from build123d import *

# Parameters (mm, degrees)
F2_R     = 0.4
F3_SIZE2 = 0.3
F3_SIZE  = 1


with BuildPart() as f1:
    # F0 (on Right) → F1 (revolve)
    with BuildSketch(Plane.YZ):
        Polygon((1.5, 15.5), (0, 15.5), (0, 10), (16.5, 10), (16.5, 11.5), (1.5, 11.5), align=None)
    revolve(axis=Axis((0, 9.5578194596, 0), (0, 1, 0)))

    # F2
    f2_edges = [f1.edges().sort_by_distance(p)[0] for p in [
        (0, 0, -10),
    ]]
    fillet(f2_edges, radius=F2_R)

    # F3
    f3_edges = [f1.edges().sort_by_distance(p)[0] for p in [
        (0, 16.5, -11.5),
    ]]
    f3_side = f1.faces().sort_by_distance((0, 9, -11.5))[0]
    chamfer(f3_edges, length=F3_SIZE, length2=F3_SIZE2, reference=f3_side)


solid = f1.part
For this review, take the finished solid that the model builds, in its own axes (mm). Round coordinates to 2 decimals unless told otherwise and drop trailing zeros. Order: outer loops, then holes, each group sorted by start corner. A loop starts at its lowest first (then second) coordinate and runs counter-clockwise, first axis right, second up. Notation, with made-up numbers: M 44.25,6.5 L 50.25,6.5 A28 ccw 50.25,39.5 Z; hole C 21,-21 d6. An arc over 180 degrees is marked long. Use a Markdown table: item, result. Add a question column.
Item 1: Add section C-C, the plane y = 11. Give the boundary of the cut face in (x, z), then the cut area to 3 significant figures.
Item 2: Add section A-A, the plane x = 0. Give the boundary of the cut face in (y, z).
Item 3: Add section D-D, the plane z = 13. Give the boundary of the cut face in (x, y), then the cut area to 3 significant figures.
Item 4: To check wall thickness, follow line 1 along X through (y, z) = (3.75, 0); line 2 along Y through (x, z) = (4, 13.5); line 3 along Z through (x, y) = (8, 8.5). State the ranges of each line that lie inside material, in increasing order.
Item 5: Add section B-B, the plane z = 0. Give the boundary of the cut face in (x, y).
Item 6: Mouldability with a two-part tool opening along Z and no side actions: class faces 1 (the flat face through (12, 1.5, 0)), 2 (the cylindrical face through (11.4, 8.4, -1.5)), 3 (the cylindrical face through (-9.76, 8.56, -2.17)) as released by +Z, released by -Z, zero draft, split by the parting line, or undercut.
Item 7: Insertion check: pin 1 (3 mm diameter, centred on y = 8, z = -2.5, fed in from -X); pin 2 (8 mm diameter, centred on x = 1.5, z = -5, fed in from +Y); pin 3 (1 mm diameter, centred on y = 4, z = -7, fed in from -X); pin 4 (5 mm diameter, centred on x = 1.5, y = 9, fed in from -Z). Each pin has a flat end and moves straight along its axis. Give the tip position at first contact, or say it passes through.
Geometry results:
| question | item | result |
|---|---|---|
| 1 | outline | C 0,0 d23; hole C 0,0 d20 |
| 1 | area | 101 mm² |
| 2 | outline | M 0,-15.5 L 1.5,-15.5 L 1.5,-11.5 L 15.5,-11.5 L 16.5,-11.2 L 16.5,-10 L 0.4,-10 A0.4 ccw 0,-10.4 Z; M 0,10.4 A0.4 ccw 0.4,10 L 16.5,10 L 16.5,11.2 L 15.5,11.5 L 1.5,11.5 L 1.5,15.5 L 0,15.5 Z |
| 3 | outline | M -8.44,0 L 8.44,0 L 8.44,1.5 L -8.44,1.5 Z |
| 3 | area | 25.3 mm² |
| 4 | line 1 | x = -11.5 to -10, 10 to 11.5 |
| 4 | line 2 | y = 0 to 1.5 |
| 4 | line 3 | z = -8.26 to -6, 6 to 8.26 |
| 5 | outline | M -15.5,0 L -10.4,0 A0.4 ccw -10,0.4 L -10,16.5 L -11.2,16.5 L -11.5,15.5 L -11.5,1.5 L -15.5,1.5 Z; M 10,0.4 A0.4 ccw 10.4,0 L 15.5,0 L 15.5,1.5 L 11.5,1.5 L 11.5,15.5 L 11.2,16.5 L 10,16.5 Z |
| 6 | face 1 | zero draft |
| 6 | face 2 | split by the parting line |
| 6 | face 3 | undercut |
| 7 | pin 1 | stops at x = -11.46 |
| 7 | pin 2 | passes through |
| 7 | pin 3 | stops at x = -9.49 |
| 7 | pin 4 | stops at z = -11.5 |
